Can you work these out from the model? Positions are in its coordinate system, mm. Face numbers are marked on the shaded views. Give positions to 0.01 mm unless a question says otherwise; leave off trailing zeros. Write each loop counter-clockwise with the first axis right and the second up, starting at its lowest first coordinate (ties: lowest second). Pieces come first, ordered by that corner, then holes. Notation, with made-up numbers: (10, 62) -> (56, 62) arc R30 ccw to (56, 85) -> close; hole circle Ø5 at (26, 73.5). An arc over 180 degrees is marked (long way). Answer as CSV lines item,"result". Start each with the question number.
1. If we section it at A-A on x = 0: Write out the boundary of the cut face in (y, z), plus the area to 3 significant figures.
2. I need wall thicknesses on line 1 (X direction, y = 15.25, z = 0); line 2 (Z direction, x = -1, y = 18.5); line 3 (X direction, y = 15.25, z = 0.5). Which ranges of each line are inside material? Lowest first, please. Write a range as [from, to].
3. If we section it at C-C on z = 1.75: Write out the boundary of the cut face in (x, y), plus the area to 3 significant figures.
4. If we mould it in two halves opening along Z, with no side actions, what happens to the marked faces 1, 2, 3 and 4? For each: pulls with the +Z half, pulls with the -Z half, needs draft (parallel to the pull), parting line crosses it, or undercut.
5. If we section it at B-B on y = 16.75: Write out the boundary of the cut face in (x, z).
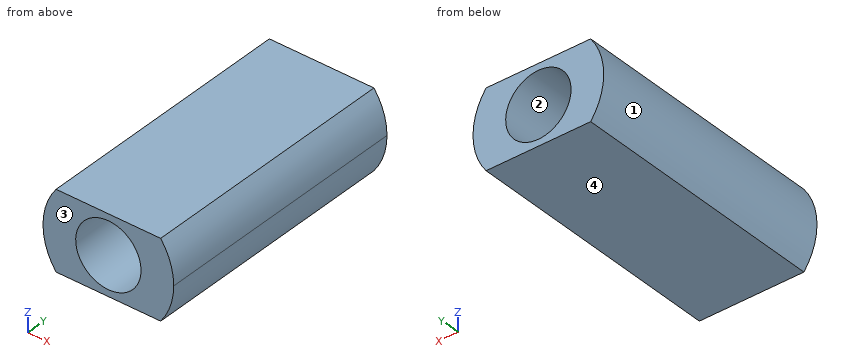
```python
from build123d import *

# Parameters (mm, degrees)
SCHIZZO1_W                   = 8
SCHIZZO1_H                   = 6
ESTRUSIONE_ESTRUSIONE1_DEPTH = 20
SCHIZZO2_R                   = 2.5
TAGLIO_ESTRUSIONE1_DEPTH     = 20


with BuildPart() as part:
    # Schizzo1 → Estrusione-Estrusione1 (new body)
    with BuildSketch(Plane(origin=(0, 0, 0), x_dir=(1, 0, 0), z_dir=(0, 1, 0))):
        with BuildLine():
            Line((-4, -3), (-4, 3))
            ThreePointArc((-4, 3), (-5, 0), (-4, -3))
        make_face()
        Rectangle(SCHIZZO1_W, SCHIZZO1_H)
        with BuildLine():
            ThreePointArc((5, 0), (4.74341649, 1.58113883), (4, 3))
            Line((4, 3), (4, -3))
            ThreePointArc((4, -3), (4.74341649, -1.58113883), (5, 0))
        make_face()
    extrude(amount=ESTRUSIONE_ESTRUSIONE1_DEPTH)

    # Schizzo2 → Taglio-Estrusione1 (cut)
    with BuildSketch(Plane(origin=(0, 20, 0), x_dir=(1, 0, 0), z_dir=(0, 1, 0))):
        with Locations(Location((0, 0, 0), (0, 0, 270))):
            Circle(SCHIZZO2_R)
    extrude(amount=-TAGLIO_ESTRUSIONE1_DEPTH, mode=Mode.SUBTRACT)


solid = part.part
```
Computed values:
1,outline,"(0, -3) -> (20, -3) -> (20, -2.5) -> (0, -2.5) -> close; (0, 2.5) -> (20, 2.5) -> (20, 3) -> (0, 3) -> close"
1,area,"20.0 mm2"
2,line 1,"x = [-5, -2.5], [2.5, 5]"
2,line 2,"z = [-3, -2.29], [2.29, 3]"
2,line 3,"x = [-4.97, -2.45], [2.45, 4.97]"
3,outline,"(-4.68, 0) -> (-1.79, 0) -> (-1.79, 20) -> (-4.68, 20) -> close; (1.79, 0) -> (4.68, 0) -> (4.68, 20) -> (1.79, 20) -> close"
3,area,"116 mm2"
4,face 1,"parting line crosses it"
4,face 2,"undercut"
4,face 3,"needs draft"
4,face 4,"pulls with the -Z half"
5,outline,"(-4, -3) -> (4, -3) arc R5 ccw to (4, 3) -> (-4, 3) arc R5 ccw to start; hole circle Ø5 at (0, 0)"
